CAD build for the part. Positions are in the model's coordinates, mm. Face numbers are marked on the shaded views. Coordinates: 2 decimals unless noted, no trailing zeros. Order: outer loops, then holes, each group sorted by start corner. A loop starts at its lowest first (then second) coordinate and runs counter-clockwise, first axis right, second up. Notation, with made-up numbers: (63.25, -33.5) - (89.25, -33.5) arc R15 cw to (89.25, -24.5) - close; hole circle Ø4 at (22.25, -7). An arc over 180 degrees is marked (long way). Write each question's results on one line, items separated by ' | '. Start each with the question number.
Q1. Band-saw the part on B-B, the plane x = 17. Write the cut outline in (y, z), then the cut area to 3 significant figures.
Q2. Band-saw the part on C-C, the plane y = -3.5. Write the cut outline in (x, z).
Q3. Wall check: probe 1 along X at (y, z) = (-25.5, 10.25); probe 2 along X at (y, z) = (1.5, 21.5); probe 3 along X at (y, z) = (16.5, 13.75). Give the ranges that are in metal, low to high.
Q4. Pin check, flat tips, straight feed: P1, Ø8, axis at x = -23.5, z = 4, coming from the -Y side; P2, Ø5, axis at x = -20.5, z = 22.5, coming from the +Y side; P3, Ø8, axis at x = 14.5, z = 19.5, coming from the +Y side. Stop position of each tip, or through.
Q5. Pull direction Y, two halves, no side cores. Call the marked faces 1, 2 and 3: released by +Y, released by -Y, zero draft, split by the parting line, or undercut.
```python
from build123d import *

# Parameters (mm, degrees)
F1_DEPTH = 25


with BuildPart() as f1:
    # F0 (on Top) → F1 (new body)
    with BuildSketch(Plane.XY):
        with BuildLine():
            ThreePointArc((29.995626, -0.512264), (29.998907, -0.256141), (30, 0))
            ThreePointArc((30, 0), (29.888092, 2.588808), (29.553205, 5.158303))
            ThreePointArc((29.553205, 5.158303), (23.571681, 8.329218), (26.233106, 14.55418))
            ThreePointArc((26.233106, 14.55418), (24.735282, 16.975448), (23.014675, 19.243824))
            ThreePointArc((23.014675, 19.243824), (16.249065, 18.999155), (15.441446, 25.720842))
            ThreePointArc((15.441446, 25.720842), (12.933658, 27.06881), (10.309381, 28.172978))
            ThreePointArc((10.309381, 28.172978), (4.572526, 24.578283), (0.512264, 29.995626))
            ThreePointArc((0.512264, 29.995626), (-2.333528, 29.909106), (-5.158303, 29.553205))
            ThreePointArc((-5.158303, 29.553205), (-8.329218, 23.571681), (-14.55418, 26.233106))
            ThreePointArc((-14.55418, 26.233106), (-16.975448, 24.735282), (-19.243824, 23.014675))
            ThreePointArc((-19.243824, 23.014675), (-18.17428, 21.39943), (-17.798986, 19.498878))
            ThreePointArc((-17.798986, 19.498878), (-20.519653, 15.048638), (-25.720842, 15.441446))
            ThreePointArc((-25.720842, 15.441446), (-27.06881, 12.933658), (-28.172978, 10.309381))
            ThreePointArc((-28.172978, 10.309381), (-25.518716, 8.519785), (-24.49394, 5.487031))
            ThreePointArc((-24.49394, 5.487031), (-26.140466, 1.778363), (-29.995626, 0.512264))
            ThreePointArc((-29.995626, 0.512264), (-29.909106, -2.333528), (-29.553205, -5.158303))
            ThreePointArc((-29.553205, -5.158303), (-25.23118, -6.036783), (-23.286017, -9.995062))
            ThreePointArc((-23.286017, -9.995062), (-24.086936, -12.709417), (-26.233106, -14.55418))
            ThreePointArc((-26.233106, -14.55418), (-24.735282, -16.975448), (-23.014675, -19.243824))
            ThreePointArc((-23.014675, -19.243824), (-17.57261, -18.184932), (-14.498878, -22.798986))
            ThreePointArc((-14.498878, -22.798986), (-14.740351, -24.334049), (-15.441446, -25.720842))
            ThreePointArc((-15.441446, -25.720842), (-12.933658, -27.06881), (-10.309381, -28.172978))
            ThreePointArc((-10.309381, -28.172978), (-4.820604, -24.538551), (-0.487031, -29.49394))
            ThreePointArc((-0.487031, -29.49394), (-0.493343, -29.7451), (-0.512264, -29.995626))
            ThreePointArc((-0.512264, -29.995626), (2.333528, -29.909106), (5.158303, -29.553205))
            ThreePointArc((5.158303, -29.553205), (8.329218, -23.571681), (14.55418, -26.233106))
            ThreePointArc((14.55418, -26.233106), (16.975448, -24.735282), (19.243824, -23.014675))
            ThreePointArc((19.243824, -23.014675), (18.999155, -16.249065), (25.720842, -15.441446))
            ThreePointArc((25.720842, -15.441446), (27.06881, -12.933658), (28.172978, -10.309381))
            ThreePointArc((28.172978, -10.309381), (24.578283, -4.572526), (29.995626, -0.512264))
        make_face()
    extrude(amount=F1_DEPTH)


solid = f1.part
```
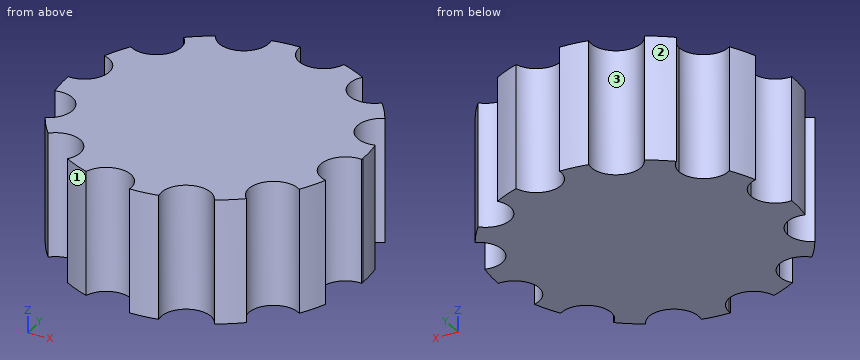
Results below:
1) outline: (-24.72, 0) - (18.47, 0) - (18.47, 25) - (-24.72, 25) - close | area: 1,080 mm²
2) outline: (-29.8, 0) - (24.91, 0) - (24.91, 25) - (-29.8, 25) - close
3) probe 1: x = -15.29 to -8.5, -2.48 to 5.84, 14.15 to 15.8 | probe 2: x = -26.48 to 29.96 | probe 3: x = -18.8 to 25.05
4) P1: stops at y = -19.24 | P2: stops at y = 24 | P3: stops at y = 28.1
5) face 1: released by -Y | face 2: released by +Y | face 3: undercut
